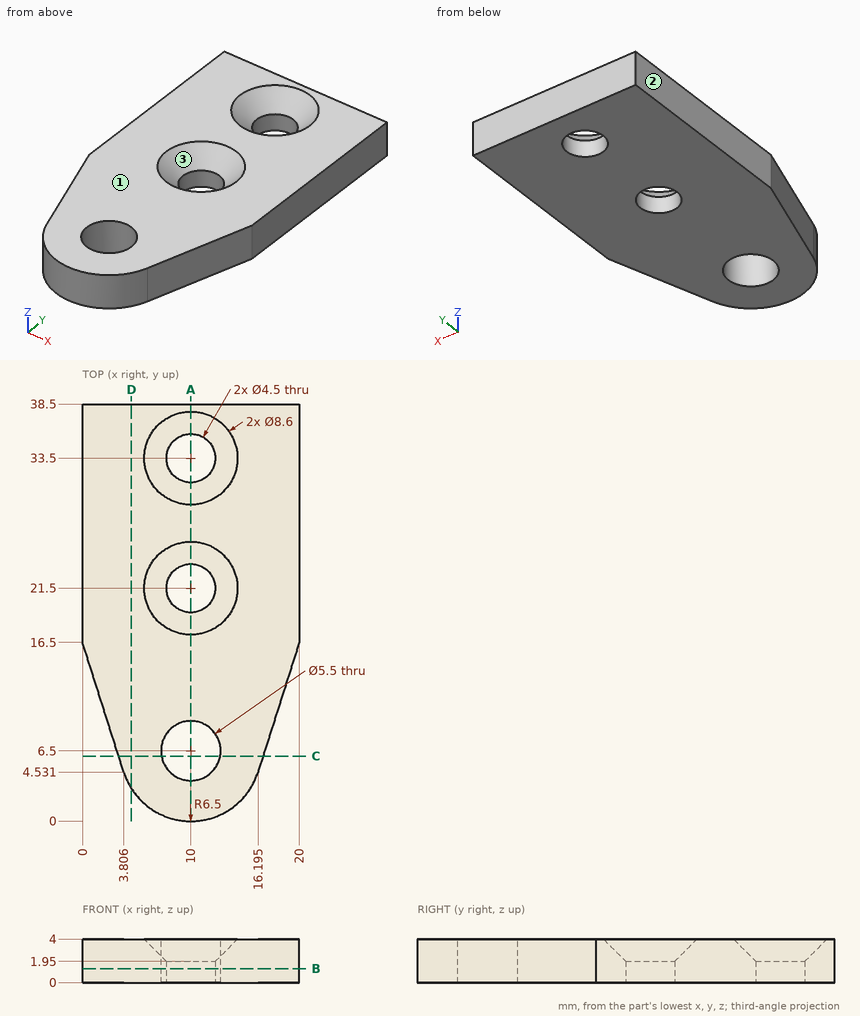
Answer from the drawing. Dimensions are ordinates in mm from the lowest x, y and z of the part. Round coordinates to 2 decimals unless told otherwise and drop trailing zeros. Loops run counter-clockwise (first coordinate to the right, second up) from the corner with the lowest first, then second, coordinate; pieces in that order, holes last.
(1) The part is cut by section C-C, the plane y = 6. Give the vertices of the cut face in (x, z) (1 decimal).
Computed values:
outline: (3.3, 0) - (7.3, 0) - (7.3, 4) - (3.3, 4) - close; (12.7, 0) - (16.7, 0) - (16.7, 4) - (12.7, 4) - close
(2) Find the intervals of material crossed by L1, parallel to X at y = 20.5, z = 2.25 (1 decimal); L2, parallel to X at y = 20, z = 1.5 (1 decimal); L3, parallel to Y at x = 9.75, z = 0.55 (1 decimal), in increasing order.
Computed values:
L1: x = 0 to 7.7, 12.3 to 20
L2: x = 0 to 8.3, 11.7 to 20
L3: y = 0 to 3.8, 9.2 to 19.3, 23.7 to 31.3, 35.7 to 38.5
(3) The part is cut by section B-B, the plane z = 1.3. Give the number of separate pieces and of enclosed holes in the cut face.
Computed values:
separate pieces: 1
enclosed holes: 3
(4) Each of these flat-tipped pins is pushed along its axis until it touches: P1, Ø3.5, axis at x = 10, y = 21.5, coming from the -Z side; P2, Ø4, axis at x = 18, y = 19, coming from the -Z side; P3, Ø1.5, axis at x = 10.5, y = 19.5, coming from the +Z side. Where does it stop, or does it pass through?
Computed values:
P1: passes through
P2: stops at z = 0
P3: stops at z = 2.51
(5) The part is cut by section A-A, the plane x = 10. Give the vertices of the cut face in (y, z).
Computed values:
outline: (0, 0) - (3.75, 0) - (3.75, 4) - (0, 4) - close; (9.25, 0) - (19.25, 0) - (19.25, 1.95) - (17.2, 4) - (9.25, 4) - close; (23.75, 0) - (31.25, 0) - (31.25, 1.95) - (29.2, 4) - (25.8, 4) - (23.75, 1.95) - close; (35.75, 0) - (38.5, 0) - (38.5, 4) - (37.8, 4) - (35.75, 1.95) - close
(6) The mould has two halves that part along X. Classify the marked faces 1, 2 and 3: pulls with the +X half, pulls with the -X half, needs draft (parallel to the pull), parting line crosses it, or undercut.
Computed values:
face 1: needs draft
face 2: pulls with the -X half
face 3: undercut
(7) The part is cut by section D-D, the plane x = 4.5. Give the vertices of the cut face in (y, z) (1 decimal), and give its area (3 significant figures).
Computed values:
outline: (3, 0) - (38.5, 0) - (38.5, 4) - (3, 4) - close
area: 142 mm2
